from build123d import *

# Parameters (mm, degrees)
SKETCH1_R           = 7.5
BOSS_EXTRUDE1_DEPTH = 1
CHAMFER1_SIZE       = 0.5
CHAMFER1_SIZE2      = 0.866025404
SKETCH2_R           = 3
CUT_EXTRUDE1_DEPTH  = 1


with BuildPart() as part:
    # Sketch1 → Boss-Extrude1 (new body)
    with BuildSketch(Plane(origin=(0, 0, 0), x_dir=(1, 0, 0), z_dir=(0, 1, 0))):
        Circle(SKETCH1_R)
    extrude(amount=BOSS_EXTRUDE1_DEPTH)

    # Chamfer1
    chamfer1_edges = [part.edges().sort_by_distance(p)[0] for p in [
        (-7.5, 1, 0),
    ]]
    chamfer1_side = [part.faces().sort_by_distance(p)[0] for p in [
        (-7.5, 0.5, 0),
    ]]
    chamfer(chamfer1_edges, length=CHAMFER1_SIZE, length2=CHAMFER1_SIZE2, reference=chamfer1_side[0])

    # Sketch2 → Cut-Extrude1 (cut)
    with BuildSketch(Plane(origin=(0, 1, 0), x_dir=(1, 0, 0), z_dir=(0, 1, 0))):
        Circle(SKETCH2_R)
    extrude(amount=-CUT_EXTRUDE1_DEPTH, mode=Mode.SUBTRACT)


solid = part.part
Read the model definition and answer for the solid it produces. Units are mm, in the model's axes. Coordinates: 2 decimals unless noted, no trailing zeros. Write each loop counter-clockwise with the first axis right and the second up, starting at its lowest first coordinate (ties: lowest second). Pieces come first, ordered by that corner, then holes. Notation, with made-up numbers: (-10.5, 72.25) -> (5.5, 72.25) arc R15 ccw to (5.5, 93.25) -> close; hole circle Ø6 at (62, 68). An arc over 180 degrees is marked (long way). Return JSON: item names as keys, results as strings.
(1) The part is cut by section A-A on x = 0. Give the vertices of the cut face in (y, z), then the cut area to 3 significant figures.
Answers below:
{"outline": "(0, -7.5) -> (0.5, -7.5) -> (1, -6.63) -> (1, -3) -> (0, -3) -> close; (0, 3) -> (1, 3) -> (1, 6.63) -> (0.5, 7.5) -> (0, 7.5) -> close", "area": "8.57 mm^2"}
(2) The part is cut by section C-C on y = 0.7. Give the vertices of the cut face in (x, z), then the cut area to 3 significant figures.
Answers below:
{"outline": "circle Ø14.31 at (0, 0); hole circle Ø6 at (0, 0)", "area": "132 mm^2"}
(3) Consider line 1 along X through (y, z) = (0.6, 0); line 2 along X through (y, z) = (0.8, 0). Determine where each line is inside the solid, lowest interval first. Write a range as from..to.
Answers below:
{"line 1": "-7.33..-3, 3..7.33", "line 2": "-6.98..-3, 3..6.98"}
(4) For a pull along X with two mould halves and no side action, classify faces 1 (the cylindrical face through (-7.493, 0.246, -0.33)), 2 (the flat face through (3.2, 0, -0.1)), 3 (the cylindrical face through (-3, 0.5, -0.1)) as pulls with the +X half, pulls with the -X half, needs draft (parallel to the pull), parting line crosses it, or undercut.
Answers below:
{"face 1": "parting line crosses it", "face 2": "needs draft", "face 3": "undercut"}
(5) The part is cut by section B-B on z = 0. Give the vertices of the cut face in (x, y), then the cut area to 3 significant figures.
Answers below:
{"outline": "(-7.5, 0) -> (-3, 0) -> (-3, 1) -> (-6.63, 1) -> (-7.5, 0.5) -> close; (3, 0) -> (7.5, 0) -> (7.5, 0.5) -> (6.63, 1) -> (3, 1) -> close", "area": "8.57 mm^2"}
(6) This flat-tipped pin is pushed along its axis until it touches: P1, Ø5, axis at x = 5, z = -2.5, coming from the -Y side. Where does it stop, or does it pass through?
Answers below:
{"P1": "y = 0"}
